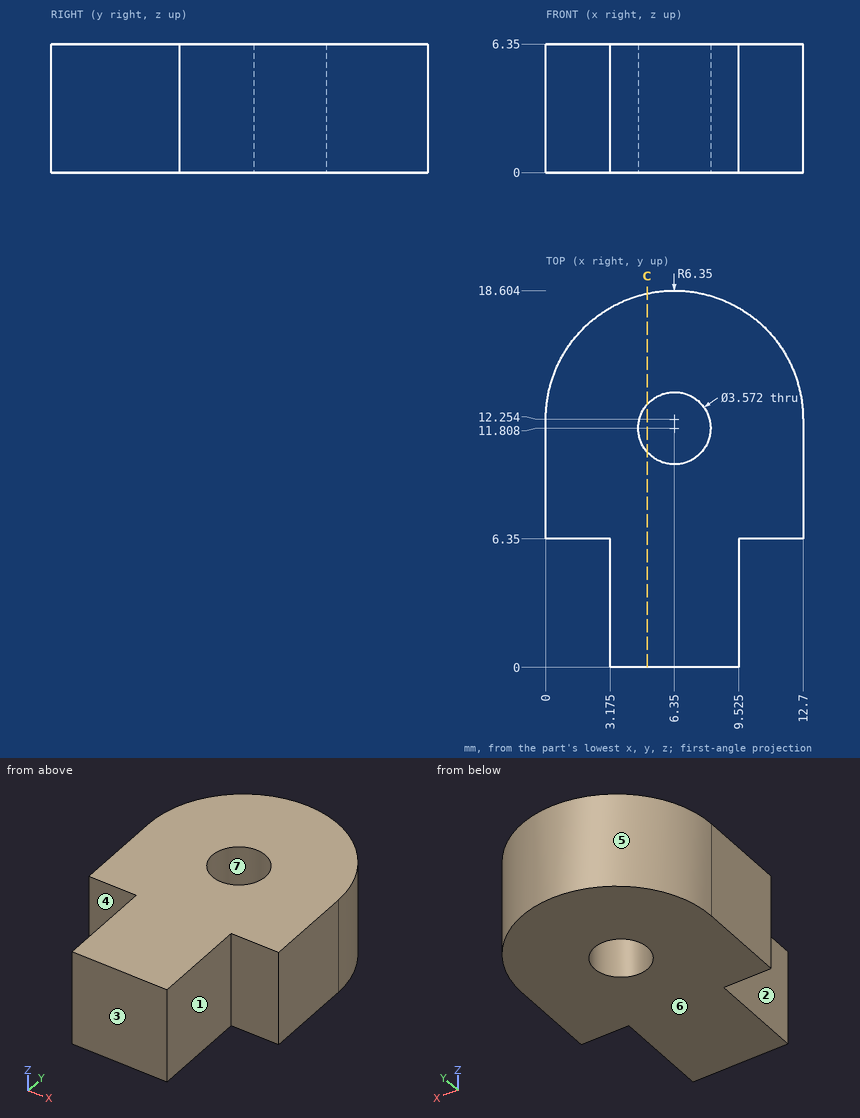
Study the drawing (mm; zero at the part's minimum x, y, z) and answer. A direction names the side the tool comes from. Give positions to 0.01 mm unless a question says otherwise; leave off trailing zeros. Write each loop counter-clockwise with the first axis right and the second up, starting at its lowest first coordinate (ties: lowest second). Pieces come first, ordered by that corner, then holes. Notation, with made-up numbers: (69, -23) -> (94, -23) arc R3 ccw to (94, -18) -> close; hole circle Ø8 at (-2, 28). An arc over 180 degrees is marked (long way). Write item = value, one per line. Start each with the question number.
1) Each of these flat-tipped pins is pushed along its axis until it touches: pin 1 (3 mm diameter, centred on x = 2, z = 1.5, fed in from +Y); pin 2 (3 mm diameter, centred on x = 6.35, y = 11.81, fed in from +Z); pin 3 (1.9 mm diameter, centred on y = 3.5, z = 3.5, fed in from -X) (3 decimals). Where does it stop, or does it pass through?
2) The part is cut by section C-C, the plane x = 5. Determine the outline of the cut face in (y, z).
3) Straight lines are drawn through the part: line 1 along Y through (x, z) = (6.35, 4.5) (1 decimal); line 2 along X through (y, z) = (10.5, 3) (1 decimal); line 3 along X through (y, z) = (4, 5.25) (1 decimal). For each, find the intervals that lie inside material, in ascending order.
4) Determine the mould class of the marked faces 4, 5, 6 and 7 for opening direction Y: +Y half, -Y half, draft (parallel to the pull), parting line (faces both ways), or undercut.
5) Which of the six approach directions +Z, -Z, +X, -X, +Y, -Y give full straight-line access (tool end or side, diameter ignored) to the marked faces 1, 2 and 3?
Solutions:
q1.pin_1 = 17.93
q1.pin_2 = through
q1.pin_3 = 3.175
q2.outline = (0, 0) -> (10.64, 0) -> (10.64, 6.35) -> (0, 6.35) -> close; (12.98, 0) -> (18.46, 0) -> (18.46, 6.35) -> (12.98, 6.35) -> close
q3.line_1 = 0 to 10, 13.6 to 18.6
q3.line_2 = 0 to 5.1, 7.6 to 12.7
q3.line_3 = 3.2 to 9.5
q4.face_4 = -Y half
q4.face_5 = +Y half
q4.face_6 = draft
q4.face_7 = undercut
q5.face_1 = +Z, -Z, +X, -Y
q5.face_2 = +Z, -Z, -X, -Y
q5.face_3 = +Z, -Z, +X, -X, -Y
